```python
from build123d import *

# Parameters (mm, degrees)
EXTRUDE_1_DEPTH = 30
SKETCH_2_R      = 15
EXTRUDE_2_DEPTH = 5


with BuildPart() as part:
    # 草图1 → 凸台-拉伸1 (new body)
    with BuildSketch(Plane.XY):
        with BuildLine():
            Line((-1.5, 8), (-1.5, 4.769696007))
            ThreePointArc((-1.5, 4.769696007), (0, 5), (1.5, 4.769696007))
            Line((1.5, 4.769696007), (1.5, 8))
            Line((1.5, 8), (-1.5, 8))
        make_face()
        with BuildLine():
            Line((1.5, 0), (0, 0))
            Line((0, 0), (-1.5, 0))
            Line((-1.5, 0), (-1.5, 4.769696007))
            ThreePointArc((-1.5, 4.769696007), (-2.958039892, -4.031128874), (5, 0))
            ThreePointArc((5, 0), (4.031128874, 2.958039892), (1.5, 4.769696007))
            Line((1.5, 4.769696007), (1.5, 0))
        make_face()
        with BuildLine():
            Line((-1.5, 0), (0, 0))
            Line((0, 0), (1.5, 0))
            Line((1.5, 0), (1.5, 4.769696007))
            ThreePointArc((1.5, 4.769696007), (0, 5), (-1.5, 4.769696007))
            Line((-1.5, 4.769696007), (-1.5, 0))
        make_face()
    extrude(amount=EXTRUDE_1_DEPTH)

    # 草图2 → 凸台-拉伸2 (add)
    with BuildSketch(Plane.XY.offset(30)):
        Circle(SKETCH_2_R)
    extrude(amount=EXTRUDE_2_DEPTH)


solid = part.part
```
Can you work these out from the model? Positions are in its coordinate system, mm. A direction names the side the tool comes from. Round coordinates to 2 decimals unless told otherwise and drop trailing zeros. Loops run counter-clockwise (first coordinate to the right, second up) from the corner with the lowest first, then second, coordinate; pieces in that order, holes last. Notation, with made-up numbers: M 56.25,10 L 112.25,10 A22 cw 112.25,37 Z; hole C 28.5,58 d9. An arc over 180 degrees is marked long. Write item = value, one per line. Start each with the question number.
(1) Suppose I cut it at B-B on z = 2.5. Write out the boundary of the cut face in (x, y), plus the area to 3 significant figures.
(2) Which directions (+Z, -Z, +X, -X, +Y, -Y) give clear straight access to the entire face, cutting with the end or side of a thin tool? Please do faces 1 (the face through (0, 0, 0)), 2 (the face through (0, 8, 15)), 3 (the face through (1.5, 6, 15)), 4 (the face through (-1.5, 6, 15)).
(3) Suppose I cut it at C-C on y = 6.75. Write out the boundary of the cut face in (x, z).
(4) Suppose I cut it at D-D on z = 33.5. Write out the boundary of the cut face in (x, y), plus the area to 3 significant figures.
(5) Suppose I cut it at A-A on x = 0. Write out the boundary of the cut face in (y, z).
(6) I need wall thicknesses on line 1 along Z through (x, y) = (8, -2.25); line 2 along X through (y, z) = (0.25, 6); line 3 along X through (y, z) = (6.75, 6). Which ranges of each line are inside material? Lowest first, please.
(7) I'm going to push flat-ended pins straight in: P1, Ø0.9, axis at x = -0.5, z = 15.5, coming from the +Y side; P2, Ø4, axis at x = 9.5, y = -2.5, coming from the -Z side; P3, Ø6, axis at x = -8.5, z = 24, coming from the +Y side; P4, Ø12, axis at y = 11, z = 9.5, coming from the -X side. Where does each tip first touch, or does it pass through?
Answer block:
q1.outline = M -1.5,4.77 A5 ccw long 1.5,4.77 L 1.5,8 L -1.5,8 Z
q1.area = 87.8 mm²
q2.face_1 = -Z, +X, -X, +Y, -Y
q2.face_2 = -Z, +X, -X, +Y
q2.face_3 = -Z, +X, +Y
q2.face_4 = -Z, -X, +Y
q3.outline = M -13.4,30 L -1.5,30 L -1.5,0 L 1.5,0 L 1.5,30 L 13.4,30 L 13.4,35 L -13.4,35 Z
q4.outline = C 0,0 d30
q4.area = 707 mm²
q5.outline = M -15,30 L -5,30 L -5,0 L 8,0 L 8,30 L 15,30 L 15,35 L -15,35 Z
q6.line_1 = 30 to 35
q6.line_2 = -4.99 to 4.99
q6.line_3 = -1.5 to 1.5
q7.P1 = 8
q7.P2 = 30
q7.P3 = through
q7.P4 = -1.5
